The listing builds one solid part. Answer for the finished solid, in the listing's coordinates (mm). A direction names the side the tool comes from. Give positions to 0.01 mm unless a question says otherwise; leave off trailing zeros. Write each loop counter-clockwise with the first axis right and the second up, starting at its lowest first coordinate (ties: lowest second). Pieces come first, ordered by that corner, then holes. Notation, with made-up numbers: (7.25, 9.5) - (18.25, 9.5) arc R12 ccw to (18.25, 19.5) - close; hole circle Ø7 at (-20.75, 2.5). An arc over 180 degrees is marked (long way). Answer in a Markdown table with one row per item. Add a question column.
from build123d import *

# Parameters (mm, degrees)
SKETCH1_W           = 20
SKETCH1_H           = 40
BOSS_EXTRUDE1_DEPTH = 40
BOSS_EXTRUDE2_DEPTH = 20
CUT_EXTRUDE1_DEPTH  = 20
CUT_EXTRUDE2_DEPTH  = 20
BOSS_EXTRUDE3_DEPTH = 20
SKETCH6_W           = 20
SKETCH6_H           = 28.284271247
CUT_EXTRUDE3_DEPTH  = 20
SKETCH7_W           = 40
SKETCH7_H           = 40
CUT_EXTRUDE4_DEPTH  = 20


with BuildPart() as part:
    # Sketch1 → Boss-Extrude1 (new body)
    with BuildSketch(Plane.XY):
        with Locations((10, 20)):
            Rectangle(SKETCH1_W, SKETCH1_H)
    extrude(amount=BOSS_EXTRUDE1_DEPTH)

    # Sketch2 → Boss-Extrude2 (add)
    with BuildSketch(Plane(origin=(0, 0, 0), x_dir=(-1, 0, 0), z_dir=(0, 0, -1))):
        Polygon((0, 0), (20, 0), (0, 40), align=None)
    extrude(amount=-BOSS_EXTRUDE2_DEPTH)

    # Sketch3 → Cut-Extrude1 (cut)
    with BuildSketch(Plane(origin=(0, 0, 0), x_dir=(-1, 0, 0), z_dir=(0, 0, -1))):
        Polygon((0, 40), (-20, 20), (-20, 40), align=None)
    extrude(amount=-CUT_EXTRUDE1_DEPTH, mode=Mode.SUBTRACT)

    # Sketch4 → Cut-Extrude2 (cut)
    with BuildSketch(Plane.ZY):
        Polygon((20, 40), (40, 0), (40, 40), align=None)
    extrude(amount=-CUT_EXTRUDE2_DEPTH, mode=Mode.SUBTRACT)

    # Sketch5 → Boss-Extrude3 (add)
    with BuildSketch(Plane(origin=(-17.777777778, 8.888888889, 17.777777778), x_dir=(-0.745355992, -0.298142397, -0.596284794), z_dir=(0.666666667, -0.333333333, -0.666666667))):
        Polygon((-23.85139176, 26.83281573), (2.98142397, -8.94427191), (-23.85139176, -17.88854382), align=None)
    extrude(amount=BOSS_EXTRUDE3_DEPTH)

    # Sketch6 → Cut-Extrude3 (cut)
    with BuildSketch(Plane(origin=(20, 20, 0), x_dir=(0, 0, -1), z_dir=(0.707106781, 0.707106781, 0))):
        with Locations((-10, 14.142135624)):
            Rectangle(SKETCH6_W, SKETCH6_H)
    extrude(amount=CUT_EXTRUDE3_DEPTH, mode=Mode.SUBTRACT)

    # Sketch7 → Cut-Extrude4 (cut)
    with BuildSketch(Plane.XZ):
        with Locations((0, 20)):
            Rectangle(SKETCH7_W, SKETCH7_H)
    extrude(amount=CUT_EXTRUDE4_DEPTH, mode=Mode.SUBTRACT)


solid = part.part
1. Given pin 1 Ø2 at (y, z) = (28.5, 18.5) entering from +X; pin 2 Ø1.5 at (x, y) = (-12, 19) entering from -Z; pin 3 Ø2 at (x, z) = (14.5, 8.5) entering from +Y; pin 4 Ø5 at (y, z) = (10.5, 29.5) entering from -X, each flat-ended and moving along its own axis, determine where each tip first touches the part or whether it passes through.
2. Section B-B (z = 36.5) is taken. Give the vertices of the cut face in (x, y).
3. Section D-D (y = 19) is taken. Give the vertices of the cut face in (x, z), and give its area (3 significant figures).
4. A tool of negligible diameter and unlimited length cuts with its end or side. For faces 1 (the face through (-7.918, 12.668, 25.748)), 2 (the face through (10, 30, 10)), from which of +Z, -Z, +X, -X, +Y, -Y can it reach the whole face along a straight path? Write none if from no direction.
5. Section A-A (y = 27.5) is taken. Give the vertices of the cut face in (x, z), and give its area (3 significant figures).
6. Section C-C (x = -4) is taken. Give the vertices of the cut face in (y, z).
7. Straight lines are drawn through the part: L1, parallel to Y at x = 5, z = 15.5; L2, parallel to X at y = 19, z = 8; L3, parallel to X at y = 8, z = 10.5. For each, find the intervals that lie inside material, in ascending order. Write a range as [from, to].
Geometry check:
| question | item | result |
|---|---|---|
| 1 | pin 1 | x = 12.5 |
| 1 | pin 2 | through |
| 1 | pin 3 | y = 26.5 |
| 1 | pin 4 | x = -8.05 |
| 2 | outline | (-3.5, 0) - (20, 0) - (20, 7) - (0, 7) - close |
| 3 | outline | (-10.5, 0) - (20, 0) - (20, 30.5) - (0, 30.5) - (-10.5, 20) - close |
| 3 | area | 875 mm² |
| 4 | face 1 | +Z, -X, +Y |
| 4 | face 2 | -Z, +X, +Y |
| 5 | outline | (-6.25, 0) - (12.5, 0) - (12.5, 20) - (20, 20) - (20, 26.25) - (0, 26.25) - (-6.25, 20) - close |
| 5 | area | 520 mm² |
| 6 | outline | (0, 0) - (32, 0) - (32, 20) - (0, 36) - close |
| 7 | L1 | [0, 35] |
| 7 | L2 | [-10.5, 20] |
| 7 | L3 | [-16, 20] |
